Build history of the part. All positions in model axes, mm. A direction names the side the tool comes from. Give positions to 0.01 mm unless a question says otherwise; leave off trailing zeros. Write each loop counter-clockwise with the first axis right and the second up, starting at its lowest first coordinate (ties: lowest second). Pieces come first, ordered by that corner, then holes. Notation, with made-up numbers: (37.25, 56.5) -> (80.25, 56.5) arc R6 ccw to (80.25, 61.5) -> close; hole circle Ø2 at (47, 57). An arc over 180 degrees is marked (long way). One line per question, with ' | ' between items. Start each with the question number.
(1) Band-saw the part on B-B, the plane z = 28.5. Give the cut face in (x, y).
(2) Drill centre line: probe 1 along Y at (x, z) = (19.5, 17.5). Where is it in solid material? Low to high. Write a range as from..to.
(3) Band-saw the part on C-C, the plane z = -42.5. Give the cut face in (x, y).
(4) Band-saw the part on A-A, the plane x = -24. Give the cut face in (y, z), and give its area (3 significant figures).
(5) Pull direction Z, two halves, no side cores. Call faces 1 (the flat face through (-63.762, 96.117, 42.042)), 2 (the flat face through (-70, 92.5, 42)), 3 (the flat face through (-1, 46, -50)): released by +Z, released by -Z, zero draft, split by the parting line, or undercut.
(6) Tool access for faces 4 (the flat face through (-63.762, 96.117, -42.042)), 5 (the flat face through (75, 46, 1)): list every direction of +Z, -Z, +X, -X, +Y, -Y with a clear straight run to the whole face (end or side of a thin tool).
(7) Pin check, flat tips, straight feed: P1, Ø0.6, axis at y = 93, z = 42.5, coming from the +X side; P2, Ø0.6, axis at x = -71, y = 92.5, coming from the -Z side; P3, Ø2, axis at x = 49.5, z = 18.5, coming from the +Y side. Stop position of each tip, or through.
from build123d import *

# Parameters (mm, degrees)
SKETCH1_W           = 150
SKETCH1_H           = 100
BOSS_EXTRUDE1_DEPTH = 93
FILLET1_R           = 1
SKETCH2_W           = 8
SKETCH2_H           = 8
CUT_EXTRUDE1_DEPTH  = 0.5
EXTRUDE_THIN1_START = 1
EXTRUDE_THIN1_DEPTH = 6


with BuildPart() as part:
    # Sketch1 → Boss-Extrude1 (new body)
    with BuildSketch(Plane(origin=(0, 0, 0), x_dir=(1, 0, 0), z_dir=(0, 1, 0))):
        Rectangle(SKETCH1_W, SKETCH1_H)
    extrude(amount=BOSS_EXTRUDE1_DEPTH)

    # Fillet1
    fillet1_edges = [part.edges().sort_by_distance(p)[0] for p in [
        (-75, 93, 0),
        (0, 93, 50),
        (75, 93, 0),
        (0, 0, 50),
        (-75, 0, 0),
        (0, 0, -50),
        (75, 0, 0),
        (75, 46.5, 50),
        (-75, 46.5, 50),
        (-75, 46.5, -50),
        (75, 46.5, -50),
        (0, 93, -50),
    ]]
    fillet(fillet1_edges, radius=FILLET1_R)

    # Sketch2 → Cut-Extrude1 (cut)
    with BuildSketch(Plane(origin=(0, 93, 0), x_dir=(1, 0, 0), z_dir=(0, 1, 0))):
        with Locations((-70, 42)):
            Rectangle(SKETCH2_W, SKETCH2_H)
    cut_extrude1 = extrude(amount=-CUT_EXTRUDE1_DEPTH, mode=Mode.SUBTRACT)

    # Mirror1: Cut-Extrude1 across plane
    add(cut_extrude1.mirror(Plane.XY), mode=Mode.SUBTRACT)

    # Sketch3 → Extrude-Thin1 (add)
    with BuildSketch(Plane.XY.offset(-46).offset(EXTRUDE_THIN1_START)):
        with BuildLine():
            Line((-67, 92.5), (-67, 93.879345126))
            ThreePointArc((-67, 93.879345126), (-66.850650808, 94.405076238), (-66.447213595, 94.773772317))
            Line((-66.447213595, 94.773772317), (-61, 97.497379115))
            Line((-61, 97.497379115), (-61.447213595, 98.391806306))
            Line((-61.447213595, 98.391806306), (-66.894427191, 95.668199508))
            ThreePointArc((-66.894427191, 95.668199508), (-67.701301617, 94.93080735), (-68, 93.879345126))
            Line((-68, 93.879345126), (-68, 92.5))
            Line((-68, 92.5), (-67, 92.5))
        make_face()
    extrude_thin1 = extrude(amount=EXTRUDE_THIN1_DEPTH)

    # Mirror2: Extrude-Thin1 across plane
    add(extrude_thin1.mirror(Plane.XY))


solid = part.part
Results:
1) outline: (-75, 1) arc R1 ccw to (-74, 0) -> (74, 0) arc R1 ccw to (75, 1) -> (75, 92) arc R1 ccw to (74, 93) -> (-74, 93) arc R1 ccw to (-75, 92) -> close
2) probe 1: y = 0..93
3) outline: (-75, 1) arc R1 ccw to (-74, 0) -> (74, 0) arc R1 ccw to (75, 1) -> (75, 92) arc R1 ccw to (74, 93) -> (-66, 93) -> (-66, 92.5) -> (-67, 92.5) -> (-67, 93.88) arc R1 cw to (-66.45, 94.77) -> (-61, 97.5) -> (-61.45, 98.39) -> (-66.89, 95.67) arc R2 ccw to (-68, 93.88) -> (-68, 92.5) -> (-74, 92.5) -> (-74, 93) arc R1 ccw to (-75, 92) -> close
4) outline: (0, -49) arc R1 ccw to (1, -50) -> (92, -50) arc R1 ccw to (93, -49) -> (93, 49) arc R1 ccw to (92, 50) -> (1, 50) arc R1 ccw to (0, 49) -> close | area: 9,300 mm²
5) face 1: zero draft | face 2: undercut | face 3: released by -Z
6) face 4: +Z, -Z, +X | face 5: +Z, -Z, +X, +Y, -Y
7) P1: stops at x = 74.71 | P2: stops at z = -49.98 | P3: stops at y = 93
